For this review, take the finished solid that the model builds, in its own axes (mm). Face numbers are marked on the shaded views. A direction names the side the tool comes from. Coordinates: 2 decimals unless noted, no trailing zeros. Loops run counter-clockwise (first coordinate to the right, second up) from the corner with the lowest first, then second, coordinate; pieces in that order, holes last. Notation, with made-up numbers: (13.25, 70) -> (60.25, 70) arc R13 cw to (60.25, 88) -> close; hole circle Ø8 at (38.25, -21.75). An arc over 180 degrees is marked (long way). Use a Markdown table: item, result.
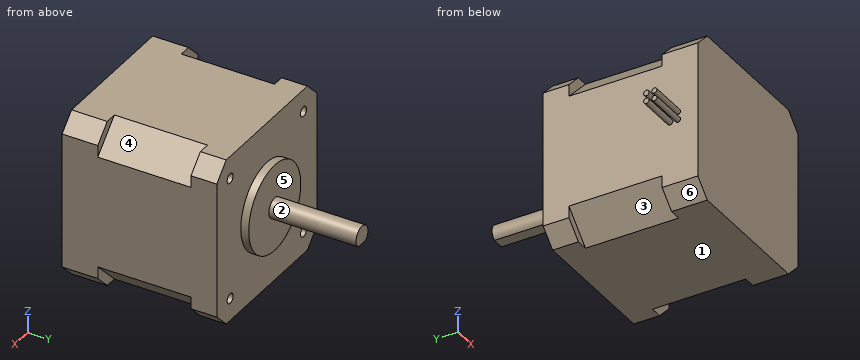
from build123d import *

# Parameters (mm, degrees)
ESQUISSE1_W                                   = 42.3
ESQUISSE1_H                                   = 42.3
BOSS_EXTRU_1_DEPTH                            = 39
ESQUISSE2_R                                   = 11
BOSS_EXTRU_2_DEPTH                            = 2
BOSS_EXTRU_3_DEPTH                            = 22
TROU_POUR_TARAUDAGE_POUR_TROU_TARAUD_M3_D     = 2.5
TROU_POUR_TARAUDAGE_POUR_TROU_TARAUD_M3_DEPTH = 4.048924226
TROU_POUR_TARAUDAGE_POUR_TROU_TARAUD_M3_TIP   = 0.751075774
CHANFREIN1_SIZE                               = 4
ENL_V_START                                   = 9
ENL_V_MAT_EXTRU_1_DEPTH                       = 23.5
ESQUISSE5_R                                   = 0.7
ESQUISSE5_R_2                                 = 0.654723083
BOSS_EXTRU_4_DEPTH                            = 10


with BuildPart() as part:
    # Esquisse1 → Boss.-Extru.1 (new body)
    with BuildSketch(Plane(origin=(0, 0, 0), x_dir=(1, 0, 0), z_dir=(0, 1, 0))):
        Rectangle(ESQUISSE1_W, ESQUISSE1_H)
    extrude(amount=BOSS_EXTRU_1_DEPTH)

    # Esquisse2 → Boss.-Extru.2 (add)
    with BuildSketch(Plane(origin=(0, 39, 0), x_dir=(1, 0, 0), z_dir=(0, 1, 0))):
        with Locations(Location((0, 0, 0), (0, 0, 270))):
            Circle(ESQUISSE2_R)
    extrude(amount=BOSS_EXTRU_2_DEPTH)

    # Esquisse3 → Boss.-Extru.3 (add)
    with BuildSketch(Plane(origin=(0, 41, 0), x_dir=(1, 0, 0), z_dir=(0, 1, 0))):
        with BuildLine():
            Line((-1.5, 2), (1.5, 2))
            ThreePointArc((1.5, 2), (0, -2.5), (-1.5, 2))
        make_face()
    extrude(amount=BOSS_EXTRU_3_DEPTH)

    # Trou pour taraudage pour trou taraudé M31
    with Locations(Plane(origin=(0, 39, 0), x_dir=(1, 0, 0), z_dir=(0, 1, 0))):
        with Locations((-15.5, 15.5), (15.5, 15.5), (15.5, -15.5), (-15.5, -15.5)):
            Hole(TROU_POUR_TARAUDAGE_POUR_TROU_TARAUD_M3_D / 2, depth=TROU_POUR_TARAUDAGE_POUR_TROU_TARAUD_M3_DEPTH)
            with Locations((0, 0, -(TROU_POUR_TARAUDAGE_POUR_TROU_TARAUD_M3_DEPTH + TROU_POUR_TARAUDAGE_POUR_TROU_TARAUD_M3_TIP / 2))):  # 118° drill point
                Cone(0, TROU_POUR_TARAUDAGE_POUR_TROU_TARAUD_M3_D / 2, TROU_POUR_TARAUDAGE_POUR_TROU_TARAUD_M3_TIP, mode=Mode.SUBTRACT)

    # Chanfrein1
    chanfrein1_edges = [part.edges().sort_by_distance(p)[0] for p in [
        (-21.15, 19.5, -21.15),
        (21.15, 19.5, -21.15),
        (21.15, 19.5, 21.15),
        (-21.15, 19.5, 21.15),
    ]]
    chamfer(chanfrein1_edges, length=CHANFREIN1_SIZE)

    # Esquisse4 → Enlèv. mat.-Extru.1 (cut)
    with BuildSketch(Plane(origin=(0, 0, 0), x_dir=(1, 0, 0), z_dir=(0, 1, 0)).offset(ENL_V_START)):
        Polygon((-14.15, 21.15), (-21.15, 14.15), (-21.15, 21.15), align=None)
        Polygon((21.15, 21.15), (14.15, 21.15), (21.15, 14.15), align=None)
        Polygon((14.15, -21.15), (21.15, -14.15), (21.15, -21.15), align=None)
        Polygon((-21.15, -21.15), (-14.15, -21.15), (-21.15, -14.15), align=None)
    extrude(amount=ENL_V_MAT_EXTRU_1_DEPTH, mode=Mode.SUBTRACT)

    # Esquisse5 → Boss.-Extru.4 (add)
    with BuildSketch(Plane.ZY.offset(21.15)):
        with Locations(Location((-1, 7, 0), (0, 0, 180))):
            Circle(ESQUISSE5_R)
        with Locations(Location((-1, 5, 0), (0, 0, 180))):
            Circle(ESQUISSE5_R_2)
        with Locations(Location((1, 5, 0), (0, 0, 180))):
            Circle(ESQUISSE5_R_2)
        with Locations(Location((1, 7, 0), (0, 0, 180))):
            Circle(ESQUISSE5_R)
    extrude(amount=BOSS_EXTRU_4_DEPTH)


solid = part.part
(1) Mouldability with a two-part tool opening along Y and no side actions: class the marked faces 4, 5 and 6 as pulls with the +Y half, pulls with the -Y half, needs draft (parallel to the pull), parting line crosses it, or undercut.
Found:
| item | result |
|---|---|
| face 4 | undercut |
| face 5 | pulls with the +Y half |
| face 6 | needs draft |
(2) For line 1 along Z through (x, y) = (-15.5, 37.3); line 2 along X through (y, z) = (36, -15), list the stretches that pass through material, from the lowest coordinate up.
Found:
| item | result |
|---|---|
| line 1 | z = -21.15 to -16.75, -14.25 to 14.25, 16.75 to 21.15 |
| line 2 | x = -21.15 to -16.65, -14.35 to 14.35, 16.65 to 21.15 |
(3) Take a section at C-C on x = -23.5. Write out the cut boundary in (y, z).
Found:
| item | result |
|---|---|
| outline | circle Ø1.31 at (5, -1); circle Ø1.31 at (5, 1); circle Ø1.4 at (7, -1); circle Ø1.4 at (7, 1) |
(4) Take a section at D-D on z = -5. Write out the cut boundary in (x, y).
Found:
| item | result |
|---|---|
| outline | (-21.15, 0) -> (21.15, 0) -> (21.15, 39) -> (9.8, 39) -> (9.8, 41) -> (-9.8, 41) -> (-9.8, 39) -> (-21.15, 39) -> close |
(5) For the marked faces 1, 2 and 3, list the 3-axis set-ups (+Z, -Z, +X, -X, +Y, -Y) from which the entire face can be reached by the end or side of a thin tool; tool diameter is ignored.
Found:
| item | result |
|---|---|
| face 1 | -Z, +X, -X, +Y, -Y |
| face 2 | +Y |
| face 3 | -Z, -X |
(6) For pin 1 Ø7.5 at (x, z) = (-18, -16) entering from +Y; pin 2 Ø1.5 at (x, z) = (-15.5, -15.5) entering from +Y; pin 3 Ø12 at (y, z) = (38.5, 7.5) entering from -X, all flat-tipped, find the tip position at first contact; note any pin that passes through.
Found:
| item | result |
|---|---|
| pin 1 | stops at y = 39 |
| pin 2 | stops at y = 34.65 |
| pin 3 | stops at x = -21.15 |
(7) Take a section at B-B on x = 0. Write out the cut boundary in (y, z), plus the area to 3 significant figures.
Found:
| item | result |
|---|---|
| outline | (0, -21.15) -> (39, -21.15) -> (39, -11) -> (41, -11) -> (41, -2) -> (63, -2) -> (63, 2.5) -> (41, 2.5) -> (41, 11) -> (39, 11) -> (39, 21.15) -> (0, 21.15) -> close |
| area | 1,790 mm^2 |
(8) Take a section at A-A on y = 18.5. Write out the cut boundary in (x, z).
Found:
| item | result |
|---|---|
| outline | (-21.15, -14.15) -> (-14.15, -21.15) -> (14.15, -21.15) -> (21.15, -14.15) -> (21.15, 14.15) -> (14.15, 21.15) -> (-14.15, 21.15) -> (-21.15, 14.15) -> close |
